```python
from build123d import *

# Parameters (mm, degrees)
ESBO_O2_R                  = 2.25
CORTE_EXTRUS_O2_DEPTH      = 19
ESBO_O7_R                  = 2.25
CORTE_EXTRUS_O6_DEPTH      = 3.329371528
CORTE_EXTRUS_O6_DEPTH_BACK = 20.716036402
CUT_EXTRUDE1_DEPTH         = 2.25
FILLET1_R                  = 0.5
CHAMFER1_SIZE              = 0.25
CHAMFER4_SIZE              = 0.25


with BuildPart() as part:
    # Esboço1 → Revolução1 (revolve)
    with BuildSketch(Plane.XY):
        Polygon((0, 25), (3, 25), (3, 5), (9, 5), (9, -5), (3, -5), (3, -9.5), (0, -9.5), (0, 0), align=None)
    revolve(axis=Axis((0, 0, 0), (0, 1, 0)))

    # Esboço2 → Corte-extrusão2 (cut, through all)
    with BuildSketch(Plane.ZY.offset(9)):
        Circle(ESBO_O2_R)
    extrude(amount=-CORTE_EXTRUS_O2_DEPTH, mode=Mode.SUBTRACT)

    # Esboço7 → Corte-extrusão6 (cut, two sides)
    with BuildSketch(Plane(origin=(-7.794228634, 0, 4.5), x_dir=(0.258819045, 0, 0.965925826), z_dir=(-0.965925826, 0, 0.258819045))) as corte_extrus_o6_sk:
        Circle(ESBO_O7_R)
    extrude(amount=CORTE_EXTRUS_O6_DEPTH, mode=Mode.SUBTRACT)
    extrude(corte_extrus_o6_sk.sketch, amount=-CORTE_EXTRUS_O6_DEPTH_BACK, mode=Mode.SUBTRACT)

    # Sketch1 → Cut-Extrude1 (cut, symmetric)
    with BuildSketch(Plane(origin=(0, 0, 0), x_dir=(1, 0, 0), z_dir=(0, 1, 0))):
        Polygon((9, 0), (-10.844388007, 0), (-10.42876147, -5.205920946), align=None)
    extrude(amount=CUT_EXTRUDE1_DEPTH, both=True, mode=Mode.SUBTRACT)

    # Fillet1
    fillet1_edges = [part.edges().sort_by_distance(p)[0] for p in [
        (-3, -5, 0),
        (-3, 5, 0),
    ]]
    fillet(fillet1_edges, radius=FILLET1_R)

    # Chamfer1
    chamfer1_edges = [part.edges().sort_by_distance(p)[0] for p in [
        (-3, -9.5, 0),
        (-3, 25, 0),
    ]]
    chamfer(chamfer1_edges, length=CHAMFER1_SIZE)

    # Chamfer4
    chamfer4_edges = [part.edges().sort_by_distance(p)[0] for p in [
        (-9, -5, 0),
        (-9, 5, 0),
    ]]
    chamfer(chamfer4_edges, length=CHAMFER4_SIZE)


solid = part.part
```
Build history of the part. All positions in model axes, mm. A direction names the side the tool comes from. Round coordinates to 2 decimals unless told otherwise and drop trailing zeros. Write each loop counter-clockwise with the first axis right and the second up, starting at its lowest first coordinate (ties: lowest second). Pieces come first, ordered by that corner, then holes.
1) 3-axis set-ups, long thin cutter, end or side, ignore diameter. For faces 4 (the flat face through (-2, -2.25, 2)), 5 (the cylindrical face through (-0.13, 0.05, -2.25)), 6 (the cylindrical face through (-3, 15, 0)), 7 (the flat face through (0, 25, 0)), 8 (the flat face through (0, -5, 4)): which of +Z, -Z, +X, -X, +Y, -Y reach the whole face in a straight line?
2) Band-saw the part on B-B, the plane y = -3.5. List the corners of the cut face in (x, z), and give its area (3 significant figures).
3) Drill centre lines: probe 1 along Y at (x, z) = (-4, 1); probe 2 along Y at (x, z) = (-7.75, -2.75); probe 3 along Y at (x, z) = (-1.5, 4). Where is each one in solid material? Low to high.
4) Pin check, flat tips, straight feed: pin 1 (4 mm diameter, centred on x = 0, z = -4, fed in from +Y); pin 2 (1.5 mm diameter, centred on y = -5, z = -6, fed in from +X); pin 3 (4 mm diameter, centred on x = 3.5, z = -4.5, fed in from -Y); pin 4 (1.5 mm diameter, centred on x = 7, z = -6.5, fed in from +Y). Stop position of each tip, or through.
5) Band-saw the part on C-C, the plane y = 20. List the corners of the cut face in (x, z), and give its area (3 significant figures).
6) Mould opens along Z. For faces 1 (the cylindrical face through (-3, -7, 0)), 2 (the flat face through (-2, 2.25, 2)), 3 (the flat face through (0, 5, 4)) say: +Z half, -Z half, draft (parallel to the pull), parting line (faces both ways), or undercut.
Ans:
1. face 4: -X
1. face 5: +X, -X
1. face 6: +Y
1. face 7: +Z, -Z, +X, -X, +Y
1. face 8: -Y
2. outline: circle Ø18 at (0, 0)
2. area: 254 mm2
3. probe 1: y = -5 to -2.25, 2.25 to 5
3. probe 2: y = -5 to 5
3. probe 3: y = -5 to -1.94, 1.94 to 5
4. pin 1: stops at y = 25
4. pin 2: stops at x = 7.28
4. pin 3: stops at y = -5
4. pin 4: stops at y = 4.95
5. outline: circle Ø6 at (0, 0)
5. area: 28.3 mm2
6. face 1: parting line
6. face 2: undercut
6. face 3: draft
